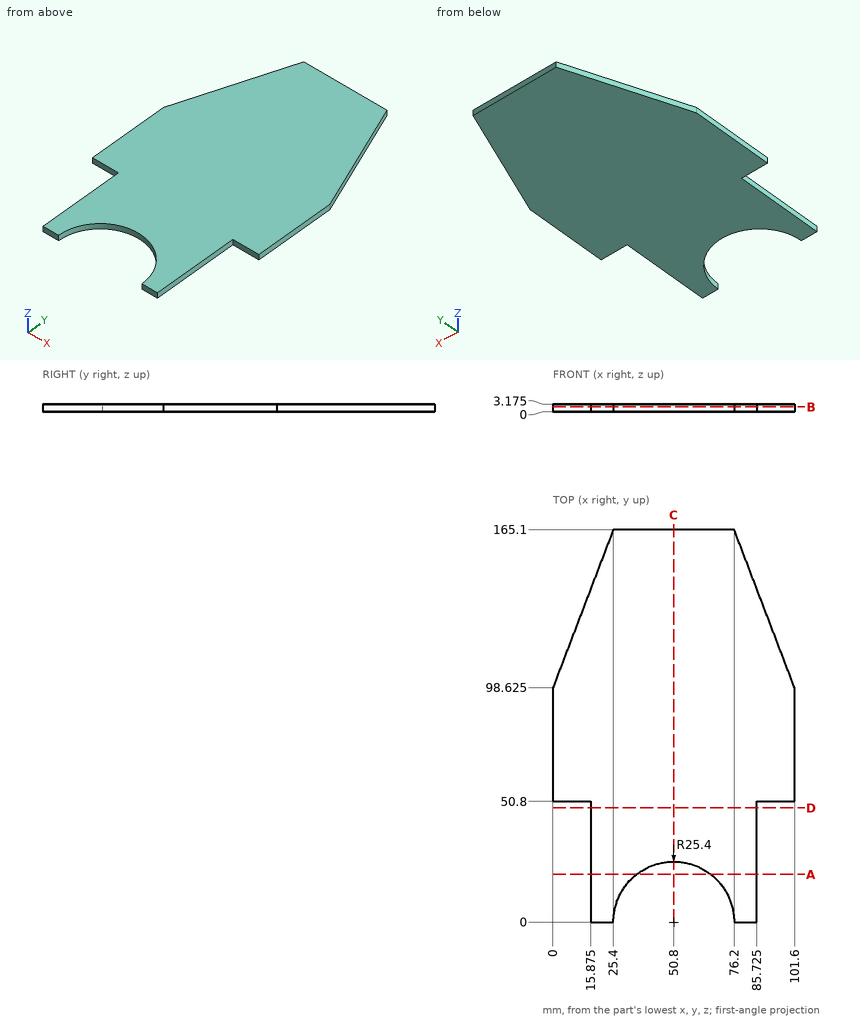
Geometry: see drawing. Coordinates: mm, zero at the bounding-box minimum. Round coordinates to 2 decimals unless told otherwise and drop trailing zeros. Write each loop counter-clockwise with the first axis right and the second up, starting at its lowest first coordinate (ties: lowest second). Pieces come first, ordered by that corner, then holes. Notation, with made-up numbers: (44, 8) - (51, 8) arc R32 ccw to (51, 43) - close; hole circle Ø5 at (57, 36). An arc over 180 degrees is marked (long way). Use CSV: the item, a comma, the result in double quotes. Start each with the question number.
(1) Cut plane A-A, the plane y = 20. Return loops of the section in (x, z) (3 decimals).
(2) Cut plane C-C, the plane x = 50.8. Return loops of the section in (y, z) (3 decimals).
(3) First-contact query: pin 1 Ø1 at (x, z) = (96, 2) entering from -Y. Flat tip, straight axial feed; report the tip coordinate or a pass-through.
(4) Material intervals for probe 1 along X at (y, z) = (11, 0.45) (3 decimals); probe 2 along Y at (x, z) = (50, 2.4); probe 3 along X at (y, z) = (49, 0.65) (3 decimals), sorted ascending. Write a range as [from, to].
(5) Cut plane D-D, the plane y = 48. Return loops of the section in (x, z) (3 decimals).
(6) Cut plane B-B, the plane z = 2. Return loops of the section in (x, y) (3 decimals), and give its area (3 significant figures).
Geometry says:
1,outline,"(15.875, 0) - (35.142, 0) - (35.142, 3.175) - (15.875, 3.175) - close; (66.458, 0) - (85.725, 0) - (85.725, 3.175) - (66.458, 3.175) - close"
2,outline,"(25.4, 0) - (165.1, 0) - (165.1, 3.175) - (25.4, 3.175) - close"
3,pin 1,"y = 50.8"
4,probe 1,"[15.875, 27.905], [73.695, 85.725]"
4,probe 2,"[25.39, 165.1]"
4,probe 3,"[15.875, 85.725]"
5,outline,"(15.875, 0) - (85.725, 0) - (85.725, 3.175) - (15.875, 3.175) - close"
6,outline,"(0, 50.8) - (15.875, 50.8) - (15.875, 0) - (25.4, 0) arc R25.4 cw to (76.2, 0) - (85.725, 0) - (85.725, 50.8) - (101.6, 50.8) - (101.6, 98.625) - (76.2, 165.1) - (25.4, 165.1) - (0, 98.625) - close"
6,area,"12,500 mm²"
